Geometry: final body of the model. Coordinates: model frame, mm. A direction names the side the tool comes from. Give positions to 0.01 mm unless a question says otherwise; leave off trailing zeros. Loops run counter-clockwise (first coordinate to the right, second up) from the corner with the lowest first, then second, coordinate; pieces in that order, holes last.
Autodesk Inventor part; units mm, degrees
ref_plane "YZ Plane" through (0, 0, 0) normal (1, 0, 0) x (0, 1, 0)
ref_plane "XZ Plane" through (0, 0, 0) normal (0, 1, 0) x (-1, 0, 0)
ref_plane "XY Plane" through (0, 0, 0) normal (0, 0, 1) x (1, 0, 0)
sketch "Sketch1" plane through (0, 0, 0) normal (0, 0, 1) x (1, 0, 0)
  line L0 (-12.7, -25.4) -> (12.7, -25.4)
  line L1 (12.7, -25.4) -> (12.7, 25.4)
  line L2 (12.7, 25.4) -> (-12.7, 25.4)
  line L3 (-12.7, 25.4) -> (-12.7, -25.4)
  line L4 (-12.7, -25.4) -> (12.7, 25.4) construction
  line L5 (12.7, -25.4) -> (-12.7, 25.4) construction
  line L6 (-11.1252, 23.8252) -> (11.1252, 23.8252)
  line L7 (11.1252, 23.8252) -> (11.1252, -23.8252)
  line L8 (11.1252, -23.8252) -> (-11.1252, -23.8252)
  line L9 (-11.1252, -23.8252) -> (-11.1252, 23.8252)
  line L10 (-11.1252, 23.8252) -> (11.1252, -23.8252) construction
  line L11 (11.1252, 23.8252) -> (-11.1252, -23.8252) construction
  point P0 (0, 0)
  dimension "d0" = 25.4
  dimension "d1" = 50.8
  dimension "d2" = 22.2504
  dimension "d3" = 47.6504
extrude "Extrusion2" add sketch "Sketch1" along normal blind 762
hole "Hole1" at (12.7, -5.08, 114.4016) direction (-1, 0, 0) diameter 28.575 depth 5.08 tip angle 118
hole "Hole2" at (12.7, -5.08, 647.5984) direction (-1, 0, 0) diameter 28.575 depth 5.08 tip angle 118
properties part number "sides" material "Aluminum 6061"
Item 1: Ray query, probe 1 along Z at (x, y) = (11.95, -5.08); probe 2 along X at (y, z) = (-15, 552); probe 3 along Y at (x, z) = (-9, 459.5). Return the intervals inside material, ascending.
Values follow:
probe 1: z = 0 to 100.11, 128.69 to 633.31, 661.89 to 762
probe 2: x = -12.7 to -11.13, 11.13 to 12.7
probe 3: y = -25.4 to -23.83, 23.83 to 25.4
Item 2: Section query A-A on x = -7. Return loops of the section in (y, z), plus the area to 3 significant figures.
Values follow:
outline: (-25.4, 0) - (-23.83, 0) - (-23.83, 762) - (-25.4, 762) - close; (23.83, 0) - (25.4, 0) - (25.4, 762) - (23.83, 762) - close
area: 2,400 mm2
Item 3: Set-up query: faces 5 (the face through (11.902, -9.372, 100.774)), 6 (the face through (0, 23.825, 376)), 7 (the face through (-11.3, 2, 0)). Return all of +Z, -Z, +X, -X, +Y, -Y with unobstructed straight access to the full face (end or side cutting, diameter ignored); none if empty.
Values follow:
face 5: +X
face 6: +Z, -Z
face 7: -Z, +X, -X, +Y, -Y
Item 4: Pin query (flat end, axial travel): pin 1 (17 mm diameter, centred on y = -5.08, z = 647.6, fed in from +X). Return the tip coordinate at first contact, or that it passes through.
Values follow:
pin 1: stops at x = -11.13
Item 5: Section query B-B on y = -5.08. Return loops of the section in (x, z).
Values follow:
outline: (-12.7, 0) - (-11.13, 0) - (-11.13, 762) - (-12.7, 762) - close; (11.13, 0) - (12.7, 0) - (12.7, 100.11) - (11.13, 100.11) - close; (11.13, 128.69) - (12.7, 128.69) - (12.7, 633.31) - (11.13, 633.31) - close; (11.13, 661.89) - (12.7, 661.89) - (12.7, 762) - (11.13, 762) - close
Item 6: Section query C-C on z = 369.5. Return loops of the section in (x, y), plus the area to 3 significant figures.
Values follow:
outline: (-12.7, -25.4) - (12.7, -25.4) - (12.7, 25.4) - (-12.7, 25.4) - close; hole (-11.13, -23.83) - (11.13, -23.83) - (11.13, 23.83) - (-11.13, 23.83) - close
area: 230 mm2
Item 7: Draft query along X for faces 1 (the face through (11.125, 0, 376)), 2 (the face through (0, 25.4, 376)), 3 (the face through (-12.7, 0, 376)), 4 (the face through (-11.125, 0, 376)). Return one class per face: +X half, -X half, draft (parallel to the pull), parting line (faces both ways), or undercut.
Values follow:
face 1: undercut
face 2: draft
face 3: -X half
face 4: undercut
